Could you check a few things on this model? Use its own coordinates, in mm. Face numbers are marked on the shaded views. A direction names the side the tool comes from. Round coordinates to 2 decimals unless told otherwise and drop trailing zeros. Loops run counter-clockwise (first coordinate to the right, second up) from the corner with the lowest first, then second, coordinate; pieces in that order, holes last. Notation, with made-up numbers: M 69,41 L 86,41 A16 ccw 86,61 Z; hole C -14.5,88 d7. An arc over 180 degrees is marked long. One line per item, written item: value. Start each with the question number.
Q1. Imagine slicing it at A-A (z = 0). Please give me the cut outline in (x, y).
Q2. Please list where these lines run through material, in increasing order: line 1 along Y through (x, z) = (5, 2); line 2 along Z through (x, y) = (0, 1.75).
Q3. Imagine slicing it at C-C (y = -1.2). Please give me the cut outline in (x, z).
Q4. Imagine slicing it at B-B (x = 0). Please give me the cut outline in (y, z).
Q5. Which directions (+Z, -Z, +X, -X, +Y, -Y) give clear straight access to the entire face, cutting with the end or side of a thin tool? Please do the marked faces 1, 2 and 3.
Q6. Imagine slicing it at D-D (z = 6.25). Please give me the cut outline in (x, y).
Q7. I'm going to push flat-ended pins straight in: pin 1 Ø1.5 at (y, z) = (0.5, -5.5) entering from -X; pin 2 Ø2 at (x, y) = (4.5, 2.5) entering from -Z; pin 3 Ø1.5 at (x, z) = (-5, 3.5) entering from -Y. Where does each tip first touch, or does it pass through?
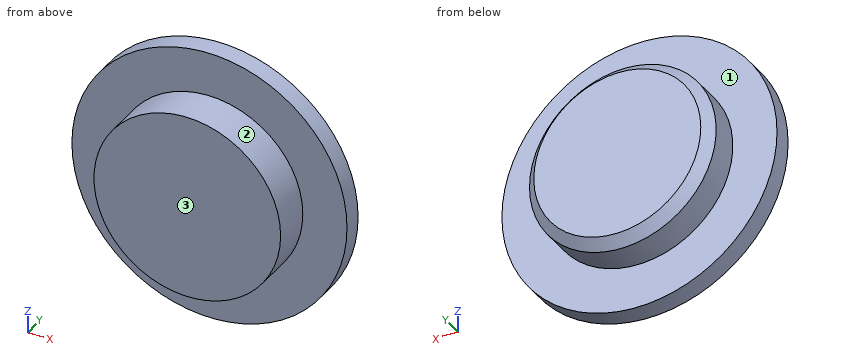
Autodesk Inventor part; units mm, degrees
ref_plane "YZ Plane" through (0, 0, 0) normal (1, 0, 0) x (0, 1, 0)
ref_plane "XZ Plane" through (0, 0, 0) normal (0, 1, 0) x (-1, 0, 0)
ref_plane "XY Plane" through (0, 0, 0) normal (0, 0, 1) x (1, 0, 0)
sketch "Sketch1" plane through (0, 0, 0) normal (0, 1, 0) x (-1, 0, 0)
  circle A0 centre (0, 0) radius 7
  dimension "d0" = 14
extrude "Extrusion1" add sketch "Sketch1" along normal blind 1
sketch "Sketch2" plane through (0, 1, 0) normal (0, 1, 0) x (1, 0, 0)
  circle A0 centre (0, 0) radius 4.75
  dimension "d3" = 9.5
extrude "Extrusion2" add sketch "Sketch2" along normal blind 2
sketch "Sketch3" plane through (0, 0, 0) normal (0, -1, 0) x (1, 0, 0)
  circle A0 centre (0, 0) radius 4.75
extrude "Extrusion3" add sketch "Sketch3" along normal blind 2
chamfer "Chamfer1" distance 0.5 angle 45 1 edges at (-4.75, 3, 0)
equation "\"BendRadius\" = Thickness"
equation "\"BendReliefWidth\" = Thickness"
equation "\"BendReliefDepth\" = 0.5 * Thickness"
equation "\"CornerReliefSize\" = 4 * Thickness"
equation "\"MinimumRemnant\" = 2 * Thickness"
equation "\"TransitionRadius\" = BendRadius"
equation "\"JacobiRadiusSize\" = BendRadius"
equation "\"GapSize\" = Thickness"
Report:
1. outline: M -7,0 L -4.75,0 L -4.75,-2 L 4.75,-2 L 4.75,0 L 7,0 L 7,1 L 4.75,1 L 4.75,2.5 L 4.25,3 L -4.25,3 L -4.75,2.5 L -4.75,1 L -7,1 Z
2. line 1: y = 0 to 1
2. line 2: z = -4.75 to 4.75
3. outline: C 0,0 d9.5
4. outline: M -2,-4.75 L 0,-4.75 L 0,-7 L 1,-7 L 1,-4.75 L 2.5,-4.75 L 3,-4.25 L 3,4.25 L 2.5,4.75 L 1,4.75 L 1,7 L 0,7 L 0,4.75 L -2,4.75 Z
5. face 1: +Y
5. face 2: -Y
5. face 3: +Z, -Z, +X, -X, -Y
6. outline: M -3.15,0 L 3.15,0 L 3.15,1 L -3.15,1 Z
7. pin 1: stops at x = -5.14
7. pin 2: stops at z = -3.21
7. pin 3: stops at y = 0
